Autodesk Fusion 360 part; units mm, degrees
sketch "Sketch1" plane through (0, 0, 0) normal (0, 1, 0) x (1, 0, 0)
  line L0 (-7, 31.5) -> (-7, 0) construction
  line L1 (-35.9586, 21.9692) -> (-30.3122, -2.5628)
  line L2 (-7, 31.5) -> (-35.9586, 21.9692)
  line L3 (-22.2116, -4.1306) -> (-17.9378, -2.5628)
  line L4 (-27.5018, 14.6711) -> (-28.4889, 18.96)
  line L5 (-26.0384, -4.1306) -> (-24.125, 0)
  line L6 (-30.3122, -2.5628) -> (-24.125, 0)
  line L7 (-24.125, 0) -> (-17.9378, -2.5628)
  line L8 (-7, 31.5) -> (-14, -20.9929)
  line L9 (-7, 31.5) -> (-34.239, 31.5)
  circle A0 centre (-24.125, -8.75) radius 5
  line L10 (-24.125, 0) -> (-27.5018, 14.6711)
  circle A1 centre (-24.125, -8.75) radius 2.5
  line L11 (-30.3122, -14.9372) -> (-32.875, -8.75)
  line L12 (-28.7444, -10.6634) -> (-32.875, -8.75)
  line L13 (-17.9378, -2.5628) -> (-15.375, -8.75)
  line L14 (-24.125, -17.5) -> (-26.0384, -13.3694)
  line L15 (-43.7102, -20.9929) -> (-14, -20.9929)
  line L16 (-19.5056, -10.6634) -> (-17.9378, -14.9372)
  line L17 (-17.9378, -14.9372) -> (-24.125, -17.5)
  line L18 (-15.375, -8.75) -> (-17.9378, -14.9372)
  line L19 (-32.875, -8.75) -> (-28.7444, -6.8366)
  line L20 (-26.0384, -13.3694) -> (-30.3122, -14.9372)
  line L21 (-19.5056, -6.8366) -> (-15.375, -8.75)
  line L22 (-22.2116, -13.3694) -> (-24.125, -17.5)
  line L23 (-17.9378, -14.9372) -> (-22.2116, -13.3694)
  line L24 (-34.239, 31.5) -> (-43.7102, -20.9929)
  line L25 (-32.875, -8.75) -> (-30.3122, -2.5628)
  line L26 (-24.125, -17.5) -> (-30.3122, -14.9372)
  line L27 (-17.9378, -2.5628) -> (-19.5056, -6.8366)
  line L28 (-15.375, -8.75) -> (-19.5056, -10.6634)
  line L29 (-30.3122, -14.9372) -> (-28.7444, -10.6634)
  line L30 (-24.125, 0) -> (-22.2116, -4.1306)
  line L31 (-7, 31.5) -> (-28.4889, 18.96)
  line L32 (-29.1989, 4.3652) -> (-29.1875, 4.3554)
  line L33 (-30.3122, -2.5628) -> (-26.0384, -4.1306)
  line L34 (-21.0314, -1.2814) -> (-24.125, -8.75) construction
  line L35 (-28.7444, -6.8366) -> (-30.3122, -2.5628)
  point P0 (-24.125, -8.75)
  point P1 (-14, 0)
  point P2 (-14, 0)
  point P3 (-14, 0)
  point P4 (-7, 0)
extrude "Extrude1" add sketch "Sketch1" along normal blind 10 contours L1 L2 L4 L6 L10 L31 | L5 L6 L33 | A0 L33 L35 | L5 A0 L30 | A0 L12 L19 | A0 | L3 A0 L27 | A0 L20 L29 | A0 L21 L28 | A0 L14 L22 | A0 L16 L23
chamfer "Chamfer3" distance 3 angle 45 1 edges at (-35.9586, 5, -21.9692)
chamfer "Chamfer4" distance 3 angle 45 1 edges at (-20.0545, 10, -27.2035)
chamfer "Chamfer5" distance 3 angle 45 2 edges at (-32.7975, 10, -8.2352) (-29.5283, 10, 4.6997)
Geometry: final body of the model. Coordinates: model frame, mm. A direction names the side the tool comes from. Give positions to 0.01 mm unless a question says otherwise; leave off trailing zeros. Loops run counter-clockwise (first coordinate to the right, second up) from the corner with the lowest first, then second, coordinate; pieces in that order, holes last. Notation, with made-up numbers: M 72,71.25 L 125,71.25 A17 cw 125,91.25 Z; hole C 15,39 d3. An arc over 180 degrees is marked long. Put each result on its own line as item: value.
1) Material intervals for L1, parallel to Z at x = -16, y = 3.25; L2, parallel to Z at x = -20.25, y = 7.25; L3, parallel to X at y = 1.5, z = 6.5, sorted ascending. Write a range as from..to.
Computed values:
L1: z = -28.54..-26.25, 8.46..9.04
L2: z = -26.88..-23.77, 3.41..14.09
L3: x = -28.87..-25.21, -23.04..-19.38
2) Cut plane A-A, the plane y = 1.5. Return the cut outline in (x, z) (3 decimals), plus the area to 3 significant figures.
Computed values:
outline: M -35.286,-19.046 L -33.109,-22.907 L -7,-31.5 L -28.489,-18.96 L -27.502,-14.671 L -24.125,0 L -22.212,4.131 L -17.938,2.563 L -19.506,6.837 L -15.375,8.75 L -19.506,10.663 L -17.938,14.937 L -22.212,13.369 L -24.125,17.5 L -26.038,13.369 L -30.312,14.937 L -28.744,10.663 L -32.875,8.75 L -28.744,6.837 L -30.312,2.563 Z; hole C -24.125,8.75 d5
area: 347 mm^2
3) Mould query, pull axis X, two halves, no side actions, for faces 1 (the flat face through (-23.62, 8.52, -24.43)), 2 (the flat face through (-18.71, 4.93, 4.67)), 3 (the flat face through (-20.105, 4.93, 3.358)). Classes: released by +X, released by -X, zero draft, split by the parting line, or undercut.
Computed values:
face 1: released by -X
face 2: released by +X
face 3: undercut
4) Cut plane B-B, the plane z = 8. Return the cut outline in (x, y), plus the area to 3 significant figures.
Computed values:
outline: M -31.26,0 L -26.51,0 L -26.51,10 L -31.26,10 Z; M -21.74,0 L -16.99,0 L -16.99,10 L -21.74,10 Z
area: 94.9 mm^2
5) Cut plane C-C, the plane x = -25. Return the cut outline in (y, z), plus the area to 3 significant figures.
Computed values:
outline: M 0,-25.58 L 7,-25.58 L 10,-22.42 L 10,-21 L 0,-21 Z; M 0,-3.8 L 10,-3.8 L 10,6.41 L 0,6.41 Z; M 0,11.09 L 10,11.09 L 10,15.61 L 0,15.61 Z
area: 188 mm^2
6) Cut plane D-D, the plane y = 7.75. Return the cut outline in (x, z) (3 decimals).
Computed values:
outline: M -34.739,-20.015 L -33.655,-21.938 L -10.103,-29.689 L -28.489,-18.96 L -27.502,-14.671 L -24.125,0 L -22.212,4.131 L -17.938,2.563 L -19.506,6.837 L -15.375,8.75 L -19.506,10.663 L -17.938,14.937 L -22.212,13.369 L -24.125,17.5 L -26.038,13.369 L -30.312,14.937 L -28.744,10.663 L -32.875,8.75 L -28.062,6.52 L -29.592,2.349 Z; hole C -24.125,8.75 d5
7) First-contact query: P1, Ø1.5, axis at y = 7, z = 0.5, coming from the -X side; P2, Ø3, axis at x = -24.125, z = 8.75, coming from the +Y side; P3, Ø2, axis at x = -27, y = 6, coming from the +Z side; P4, Ø1.5, axis at y = 2.5, z = -18.5, coming from the +X side. Flat tips, straight axial feed; report the tip coordinate or a pass-through.
Computed values:
P1: stops at x = -30.96
P2: passes through
P3: stops at z = 14.09
P4: stops at x = -27.99
8) Reachability of faces 4 (the flat face through (-29.517, 3.451, 4.73)), 5 (the flat face through (-31.463, 8.521, -9.218)), 6 (the flat face through (-17.59, 4.93, -25.32)), 7 (the flat face through (-23.2, 4.9, 2)), 8 (the flat face through (-25.07, 4.93, 15.46)) from +Z, -Z, +X, -X, +Y, -Y: full face, straight path, thin tool, end or side. Return the list, or none.
Computed values:
face 4: -X, +Y, -Y
face 5: -X, +Y
face 6: +X, +Y, -Y
face 7: +Y, -Y
face 8: +Z, +Y, -Y
